```python
from build123d import *

# Parameters (mm, degrees)
F0_R     = 11
F0_R_2   = 4
F1_DEPTH = 3.5
F2_SIZE  = 1


# Not quite as in the source:
# - a feature names something its author has since deleted; it is built from what else it names


with BuildPart() as f1:
    # F0 (on Top) → F1 (new body, symmetric)
    with BuildSketch(Plane.XY):
        with BuildLine():
            ThreePointArc((-6, 11.5325625947), (0, 13), (6, 11.5325625947))
            Line((6, 11.5325625947), (6, 25))
            ThreePointArc((6, 25), (0, 19), (-6, 25))
            Line((-6, 25), (-6, 11.5325625947))
        make_face()
        with BuildLine():
            ThreePointArc((-6.9874921777, -10.96243372), (-11.2583302492, -6.5), (-12.9874921777, -0.5701288746))
            Line((-12.9874921777, -0.5701288746), (-24.6506350946, -7.3038475773))
            ThreePointArc((-24.6506350946, -7.3038475773), (-18.6506350946, -7.3038475773), (-15.6506350946, -12.5))
            ThreePointArc((-15.6506350946, -12.5), (-16.4544826719, -15.5), (-18.6506350946, -17.6961524227))
            Line((-18.6506350946, -17.6961524227), (-6.9874921777, -10.96243372))
        make_face()
        with BuildLine():
            Line((24.6506350946, -7.3038475773), (12.9874921777, -0.5701288746))
            ThreePointArc((12.9874921777, -0.5701288746), (11.2583302492, -6.5), (6.9874921777, -10.96243372))
            Line((6.9874921777, -10.96243372), (18.6506350946, -17.6961524227))
            ThreePointArc((18.6506350946, -17.6961524227), (16.4544826719, -9.5), (24.6506350946, -7.3038475773))
        make_face()
        with BuildLine():
            ThreePointArc((12.9874921777, -0.5701288746), (12.9968726683, -0.2851330301), (13, 0))
            ThreePointArc((13, 0), (11.1130553854, 6.7453687816), (6, 11.5325625947))
            ThreePointArc((6, 11.5325625947), (0, 13), (-6, 11.5325625947))
            ThreePointArc((-6, 11.5325625947), (-11.2583302492, 6.5), (-12.9874921777, -0.5701288746))
            ThreePointArc((-12.9874921777, -0.5701288746), (-11.2583302492, -6.5), (-6.9874921777, -10.96243372))
            ThreePointArc((-6.9874921777, -10.96243372), (0, -13), (6.9874921777, -10.96243372))
            ThreePointArc((6.9874921777, -10.96243372), (11.2583302492, -6.5), (12.9874921777, -0.5701288746))
        make_face()
        Circle(F0_R, mode=Mode.SUBTRACT)
        with BuildLine():
            ThreePointArc((-6, 25), (0, 19), (6, 25))
            ThreePointArc((6, 25), (0, 31), (-6, 25))
        make_face()
        with Locations((0, 25)):
            Circle(F0_R_2, mode=Mode.SUBTRACT)
        with BuildLine():
            ThreePointArc((-15.6506350946, -12.5), (-18.6506350946, -7.3038475773), (-24.6506350946, -7.3038475773))
            ThreePointArc((-24.6506350946, -7.3038475773), (-26.8467875173, -15.5), (-18.6506350946, -17.6961524227))
            ThreePointArc((-18.6506350946, -17.6961524227), (-16.4544826719, -15.5), (-15.6506350946, -12.5))
        make_face()
        with Locations((-21.6506350946, -12.5)):
            Circle(F0_R_2, mode=Mode.SUBTRACT)
        with BuildLine():
            ThreePointArc((27.6506350946, -12.5), (26.8467875173, -9.5), (24.6506350946, -7.3038475773))
            ThreePointArc((24.6506350946, -7.3038475773), (16.4544826719, -9.5), (18.6506350946, -17.6961524227))
            ThreePointArc((18.6506350946, -17.6961524227), (24.6506350946, -17.6961524227), (27.6506350946, -12.5))
        make_face()
        with Locations((21.6506350946, -12.5)):
            Circle(F0_R_2, mode=Mode.SUBTRACT)
    extrude(amount=F1_DEPTH, both=True)

    # F2
    f2_edges = [f1.edges().sort_by_distance(p)[0] for p in [
        (-4, 25, 3.5),
        (-11, 0, 3.5),
        (-25.650635, -12.5, 3.5),
        (17.650635, -12.5, 3.5),
        (-25.650635, -12.5, -3.5),
        (-11, 0, -3.5),
        (17.650635, -12.5, -3.5),
        (-4, 25, -3.5),
    ]]
    chamfer(f2_edges, length=F2_SIZE)


solid = f1.part
```
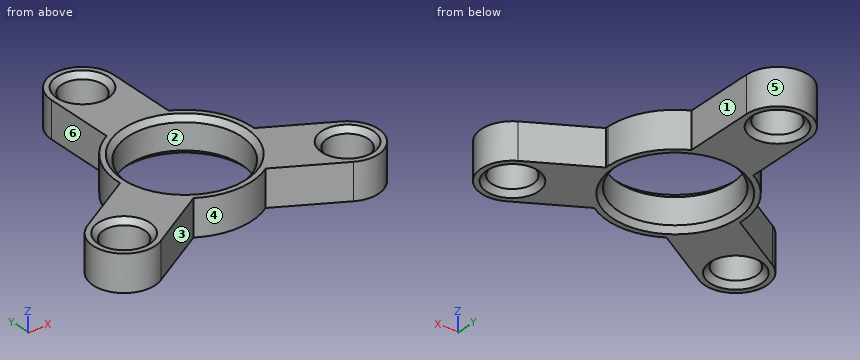
Geometry check sheet. Reference: the model listing, model coordinates, mm. Face numbers are marked on the shaded views. A direction names the side the tool comes from. Round coordinates to 2 decimals unless told otherwise and drop trailing zeros. Loops run counter-clockwise (first coordinate to the right, second up) from the corner with the lowest first, then second, coordinate; pieces in that order, holes last. Notation, with made-up numbers: M -26.75,62.25 L 7.25,62.25 A20 ccw 7.25,74.25 Z; hole C 55,21.25 d3. An arc over 180 degrees is marked long. Return JSON: item names as keys, results as strings. Group by question number.
(1) Go/stop test with flat-tipped pins: pin 1 (6.5 mm diameter, centred on x = 0, y = 25, fed in from -Z); pin 2 (2 mm diameter, centred on y = 17.5, z = 0.5, fed in from +X); pin 3 (3 mm diameter, centred on y = -2.5, z = -2.5, fed in from -X); pin 4 (4 mm diameter, centred on y = 12.5, z = -1, fed in from -X). Record where each tip stops, or that it passes through.
(2) Mould release check, pull along X, two halves, no side actions. Record for the marked faces 4, 5 and 6: pulls with the +X half, pulls with the -X half, needs draft (parallel to the pull), parting line crosses it, or undercut.
(3) Set-up check for the marked faces 1, 2 and 3: record each of +Z, -Z, +X, -X, +Y, -Y from which the full face is reachable in a straight line by a thin tool's end or side.
(4) Section check D-D, the plane x = 14.5. Enter the section's corners in (y, z).
(5) Section check A-A, the plane x = 0. Enter the section's corners in (y, z), and give its area (3 significant figures).
(6) Section check B-B, the plane z = 1.5. Enter the section's corners in (x, y), and give its area (3 significant figures).
(7) Scan lines: line 1 along Y through (x, z) = (0.5, -1); line 2 along Y through (x, z) = (1.5, -0.5); line 3 along X through (y, z) = (-14.5, 1). Record each from-to range of solid material in increasing order. Write a range as [from, to].
(8) Section check C-C, the plane y = 14.5. Enter the section's corners in (x, z), and give its area (3 significant figures).
Data:
{
 "1": {"pin 1": "through", "pin 2": "x = 6", "pin 3": "x = -18.93", "pin 4": "x = -7.66"},
 "2": {"face 4": "undercut", "face 5": "parting line crosses it", "face 6": "pulls with the -X half"},
 "3": {"face 1": "+Z, -Z, +X, +Y", "face 2": "+Z, -Z", "face 3": "+Z, -Z, -Y"},
 "4": {"outline": "M -15.3,-3.5 L -1.44,-3.5 L -1.44,3.5 L -15.3,3.5 Z"},
 "5": {"outline": "M -13,-3.5 L -12,-3.5 L -11,-2.5 L -11,2.5 L -12,3.5 L -13,3.5 Z; M 11,-2.5 L 12,-3.5 L 20,-3.5 L 21,-2.5 L 21,2.5 L 20,3.5 L 12,3.5 L 11,2.5 Z; M 29,-2.5 L 30,-3.5 L 31,-3.5 L 31,3.5 L 30,3.5 L 29,2.5 Z", "area": "94.0 mm²"},
 "6": {"outline": "M -24.65,-7.3 A6 ccw -18.65,-17.7 L -6.99,-10.96 A13 ccw 6.99,-10.96 L 18.65,-17.7 A6 ccw 24.65,-7.3 L 12.99,-0.57 A13 ccw 6,11.53 L 6,25 A6 ccw -6,25 L -6,11.53 A13 ccw -12.99,-0.57 Z; hole C -21.65,-12.5 d8; hole C 0,0 d22; hole C 0,25 d8; hole C 21.65,-12.5 d8", "area": "619 mm²"},
 "7": {"line 1": "[-12.99, -10.99], [10.99, 21.03], [28.97, 30.98]", "line 2": "[-12.91, -10.9], [10.9, 21.29], [28.71, 30.81]", "line 3": "[-27.31, -25.11], [-18.19, -13.11], [13.11, 18.19], [25.11, 27.31]"},
 "8": {"outline": "M -6,-3.5 L 6,-3.5 L 6,3.5 L -6,3.5 Z", "area": "84.0 mm²"}
}
